Verification items for the finished model (mm, model axes). Face numbers are marked on the shaded views. A direction names the side the tool comes from. Coordinates: 2 decimals unless noted, no trailing zeros. Order: outer loops, then holes, each group sorted by start corner. A loop starts at its lowest first (then second) coordinate and runs counter-clockwise, first axis right, second up. Notation, with made-up numbers: M 68.25,-31 L 120.25,-31 A29 ccw 120.25,6 Z; hole C 23.25,79 d10. An arc over 180 degrees is marked long. Answer as a JSON object with one key per item and string values. Group by question number.
(1) Cross-section at B-B (x = 0). Enter the section's corners in (y, z) (1 decimal), plus the area to 3 significant figures.
(2) Material ranges on line 1 (X direction, y = -3.5, z = 6); line 2 (X direction, y = 15, z = 7.5); line 3 (X direction, y = -8, z = 5.75), recorded low to high.
(3) Mould release check, pull along X, two halves, no side actions. Record for the marked faces 3, 4 and 5: released by +X, released by -X, zero draft, split by the parting line, or undercut.
(4) Gauge pin test, flat ends, axial feed: pin 1 Ø1.5 at (x, z) = (-3.5, 7.5) entering from +Y; pin 2 Ø4 at (x, y) = (-16.5, -9.52) entering from -Z; pin 3 Ø8 at (x, y) = (-16.5, -12.5) entering from -Z; pin 4 Ø14.5 at (x, y) = (1, -6.5) entering from +Z. Record the tip position at first contact, or that the pin passes through.
(5) Cross-section at A-A (y = 0). Enter the section's corners in (x, z) (1 decimal), plus the area to 3 significant figures.
(6) Cross-section at C-C (z = 5.25). Count the separate pieces of the cut face and the enclosed holes in it, plus the area to 3 significant figures.
(7) Cross-section at D-D (y = 18). Enter the section's corners in (x, z) (3 decimals).
(8) Access from +Z, -Z, +X, -X, +Y, -Y to the whole of each face (thin tool, end or side, straight path). Record for the marked faces 1 and 2.
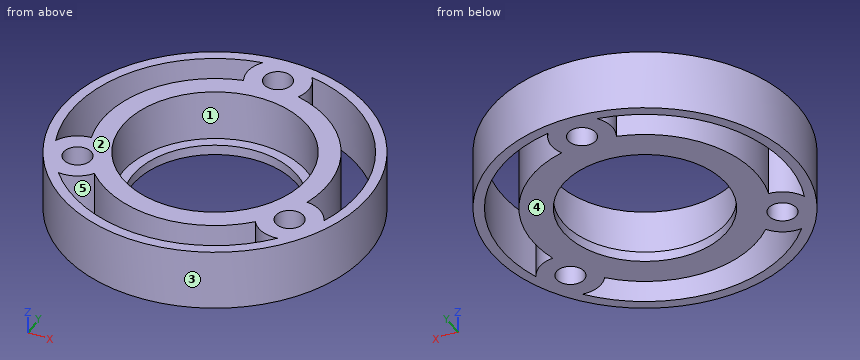
from build123d import *

# Parameters (mm, degrees)
F0_R            = 23.8125
F0_R_2          = 2.15265
F0_R_3          = 12.7
F1_DEPTH        = 9.525
F2_R            = 14.2875
F3_DEPTH        = 7.9375
F5_DEPTH        = 9.525
F5_COPIES_COUNT = 3


# Not quite as in the source:
# - a pattern or mirror of a feature is missing from the dataset's text; its kind, count and spacing are read off the source's solid


with BuildPart() as f1:
    # F0 (on Top) → F1 (new body)
    with BuildSketch(Plane.XY):
        Circle(F0_R)
        with Locations((-16.4977839421, -9.525)):
            Circle(F0_R_2, mode=Mode.SUBTRACT)
        with Locations((16.4977839421, -9.525)):
            Circle(F0_R_2, mode=Mode.SUBTRACT)
        Circle(F0_R_3, mode=Mode.SUBTRACT)
        with Locations((0, 19.05)):
            Circle(F0_R_2, mode=Mode.SUBTRACT)
    extrude(amount=F1_DEPTH)

    # F2 (on face) → F3 (cut)
    with BuildSketch(Plane.XY.offset(9.525)):
        Circle(F2_R)
    extrude(amount=-F3_DEPTH, mode=Mode.SUBTRACT)

    # F4 (on face) → F5 (cut, through all)
    with BuildSketch(Plane.XY.offset(9.525)):
        with BuildLine():
            ThreePointArc((17.0510516982, -14.2552538029), (14.4957458217, -13.8462555599), (12.5315578082, -12.1613718449))
            ThreePointArc((12.5315578082, -12.1613718449), (0, -17.4625), (-12.5315578082, -12.1613718449))
            ThreePointArc((-12.5315578082, -12.1613718449), (-14.4957458217, -13.8462555599), (-17.0510516982, -14.2552538029))
            ThreePointArc((-17.0510516982, -14.2552538029), (0, -22.225), (17.0510516982, -14.2552538029))
        make_face()
    f5 = extrude(amount=-F5_DEPTH, mode=Mode.SUBTRACT)

    # F5_copies: F5 ×3 about axis
    f5_copies_axis = Axis((0, 0, 0), (0, 0, 1))
    for i in range(1, F5_COPIES_COUNT):
        add(f5.rotate(f5_copies_axis, i * 360 / F5_COPIES_COUNT), mode=Mode.SUBTRACT)


solid = f1.part
Taken from the geometry:
{
 "1": {"outline": "M -23.8,0 L -22.2,0 L -22.2,9.5 L -23.8,9.5 Z; M -17.5,0 L -12.7,0 L -12.7,1.6 L -14.3,1.6 L -14.3,9.5 L -17.5,9.5 Z; M 12.7,0 L 16.9,0 L 16.9,9.5 L 14.3,9.5 L 14.3,1.6 L 12.7,1.6 Z; M 21.2,0 L 23.8,0 L 23.8,9.5 L 21.2,9.5 Z", "area": "100 mm²"},
 "2": {"line 1": "x = -23.55 to -21.95, -17.11 to -13.85, 13.85 to 17.11, 21.95 to 23.55", "line 2": "x = -18.49 to -16.4, -8.94 to 8.94, 16.4 to 18.49", "line 3": "x = -22.43 to -18.02, -14.98 to -11.84, 11.84 to 14.98, 18.02 to 22.43"},
 "3": {"face 3": "split by the parting line", "face 4": "zero draft", "face 5": "undercut"},
 "4": {"pin 1": "stops at y = 23.65", "pin 2": "passes through", "pin 3": "stops at z = 0", "pin 4": "stops at z = 1.59"},
 "5": {"outline": "M -23.8,0 L -22.2,0 L -22.2,9.5 L -23.8,9.5 Z; M -17.5,0 L -12.7,0 L -12.7,1.6 L -14.3,1.6 L -14.3,9.5 L -17.5,9.5 Z; M 12.7,0 L 17.5,0 L 17.5,9.5 L 14.3,9.5 L 14.3,1.6 L 12.7,1.6 Z; M 22.2,0 L 23.8,0 L 23.8,9.5 L 22.2,9.5 Z", "area": "95.8 mm²"},
 "6": {"separate pieces": "1", "enclosed holes": "7", "area": "633 mm²"},
 "7": {"outline": "M -15.59,0 L -13.037,0 L -13.037,9.525 L -15.59,9.525 Z; M -4.645,0 L -1.879,0 L -1.879,9.525 L -4.645,9.525 Z; M 1.879,0 L 4.645,0 L 4.645,9.525 L 1.879,9.525 Z; M 13.037,0 L 15.59,0 L 15.59,9.525 L 13.037,9.525 Z"},
 "8": {"face 1": "+Z", "face 2": "+Z, +X, -X, +Y, -Y"}
}
